Autodesk Inventor part; units mm, degrees
ref_plane "YZ Plane" through (0, 0, 0) normal (1, 0, 0) x (0, 1, 0)
ref_plane "XZ Plane" through (0, 0, 0) normal (0, 1, 0) x (-1, 0, 0)
ref_plane "XY Plane" through (0, 0, 0) normal (0, 0, 1) x (1, 0, 0)
sketch "Sketch1" plane through (0, 0, 0) normal (0, 1, 0) x (-1, 0, 0)
  arc A0 (27.5033, -3.6329) -> (24.5033, -6.6329) centre (27.5033, -6.6329) ccw
  arc A1 (28.5033, -3.6329) -> (28.5033, 4.3671) centre (28.5033, 0.3671) ccw
  line L0 (27.5033, -3.6329) -> (28.5033, -3.6329)
  line L1 (28.5033, 4.3671) -> (27.5033, 4.3671)
  arc A2 (24.5033, 7.3671) -> (27.5033, 4.3671) centre (27.5033, 7.3671) ccw
  line L2 (24.5033, 18.9671) -> (24.5033, 7.3671)
  line L3 (-28.2967, 18.9671) -> (24.5033, 18.9671)
  line L4 (-28.2967, 7.3671) -> (-28.2967, 18.9671)
  arc A3 (-31.2967, 4.3671) -> (-28.2967, 7.3671) centre (-31.2967, 7.3671) ccw
  line L5 (-31.2967, 4.3671) -> (-32.2967, 4.3671)
  arc A4 (-32.2967, 4.3671) -> (-32.2967, -3.6329) centre (-32.2967, 0.3671) ccw
  line L6 (-32.2967, -3.6329) -> (-31.2967, -3.6329)
  arc A5 (-28.2967, -6.6329) -> (-31.2967, -3.6329) centre (-31.2967, -6.6329) ccw
  line L7 (-28.2967, -18.2329) -> (-28.2967, -6.6329)
  line L8 (24.5033, -18.2329) -> (-28.2967, -18.2329)
  line L9 (24.5033, -6.6329) -> (24.5033, -18.2329)
  circle A6 centre (28.5033, 0.3671) radius 1.6
  circle A7 centre (-32.2967, 0.3671) radius 1.6
  circle A8 centre (-1.8967, 9.6671) radius 2.25
  circle A9 centre (15.2033, 9.6671) radius 2.25
  circle A10 centre (15.2033, -8.9329) radius 2.25
  circle A11 centre (-1.8967, -8.9329) radius 2.25
  circle A12 centre (-18.9967, -8.9329) radius 2.25
  circle A13 centre (-18.9967, 9.6671) radius 2.25
  point P0 (0, 0)
extrude "Extrusion1" add sketch "Sketch1" along normal blind 2.5
sketch "Sketch2" plane through (0, 2.5, 0) normal (0, 1, 0) x (1, 0, 0)
  line L0 (-12.6033, -12.2671) -> (-17.8033, -12.2671) construction
  line L1 (-17.8033, -12.2671) -> (-17.8033, -7.0671) construction
  line L2 (-17.8033, -7.0671) -> (-12.6033, -7.0671) construction
  line L3 (-12.6033, -7.0671) -> (-12.6033, -12.2671) construction
  circle A0 centre (-15.2033, -9.6671) radius 2.25 construction
  line L4 (-12.6033, -12.2671) -> (-17.8033, -7.0671) construction
  line L5 (-17.8033, -12.2671) -> (-12.6033, -7.0671) construction
  circle A1 centre (-17.8033, -7.0671) radius 0.75
  circle A2 centre (-12.6033, -12.2671) radius 0.75
  circle A3 centre (-17.8033, 11.5329) radius 0.75
  circle A4 centre (-12.6033, 6.3329) radius 0.75
  circle A5 centre (-0.7033, -7.0671) radius 0.75
  circle A6 centre (4.4967, -12.2671) radius 0.75
  circle A7 centre (-0.7033, 11.5329) radius 0.75
  circle A8 centre (4.4967, 6.3329) radius 0.75
  circle A9 centre (16.3967, -7.0671) radius 0.75
  circle A10 centre (21.5967, -12.2671) radius 0.75
  circle A11 centre (16.3967, 11.5329) radius 0.75
  circle A12 centre (21.5967, 6.3329) radius 0.75
  point P0 (0, 0)
  dimension "d2" = 1.5
  dimension "d3" = 1.5
  dimension "d6" = 18.6
  dimension "d9" = 17.1
  dimension "d14" = 5.2
  dimension "d15" = 5.2
extrude "Extrusion2" cut sketch "Sketch2" against normal through all
equation "\"d3\" = d2"
Design review of the part built by this model. Coordinates are the model's own, in mm. Round coordinates to 2 decimals unless told otherwise and drop trailing zeros. Order: outer loops, then holes, each group sorted by start corner. A loop starts at its lowest first (then second) coordinate and runs counter-clockwise, first axis right, second up. Notation, with made-up numbers: (-15.5, -27) - (-9.5, -27) arc R20 ccw to (-9.5, 12) - close; hole circle Ø2 at (83.25, 31). An arc over 180 degrees is marked (long way). One line per question, with ' | ' between items.
Item 1: Take a section at D-D, the plane z = -2. Write out the cut boundary in (x, y), then the cut area to 3 significant figures.
Checks:
outline: (-31.73, 0) - (35.52, 0) - (35.52, 2.5) - (-31.73, 2.5) - close | area: 168 mm²
Item 2: Take a section at B-B, the plane z = -10. Write out the cut boundary in (x, y).
Checks:
outline: (-24.5, 0) - (-17.18, 0) - (-17.18, 2.5) - (-24.5, 2.5) - close; (-13.22, 0) - (-0.08, 0) - (-0.08, 2.5) - (-13.22, 2.5) - close; (3.88, 0) - (17.02, 0) - (17.02, 2.5) - (3.88, 2.5) - close; (20.98, 0) - (28.3, 0) - (28.3, 2.5) - (20.98, 2.5) - close
Item 3: Draft analysis for pull direction Z (two halves, no side actions). For faces 1 (the face through (2, 0, 1)), 2 (the face through (29.2, 1.23, -4.49)), 3 (the face through (-12.77, 1.27, -5.6)), 4 (the face through (22.29, 1.27, -6.05)), state which applies: +Z half, -Z half, draft (parallel to the pull), parting line (faces both ways), or undercut.
Checks:
face 1: draft | face 2: -Z half | face 3: undercut | face 4: undercut
Item 4: Take a section at C-C, the plane y = 0.6. Give the number of separate pieces and of enclosed holes in the cut face, then the cut area to 3 significant figures.
Checks:
separate pieces: 1 | enclosed holes: 20 | area: 1,950 mm²
Item 5: Wall thickness on line 1 (Z direction, x = 2, y = 1.4); line 2 (X direction, y = 0.3, z = 9.5); line 3 (X direction, y = 1.5, z = 1): over which ranges is each line inside the solid? List them lowest first. Write a range as [from, to].
Checks:
line 1: [-18.23, -11.18], [-6.69, 7.42], [11.91, 18.97] | line 2: [-24.5, -17.45], [-12.96, -0.35], [4.14, 16.75], [21.24, 28.3] | line 3: [-32.45, -29.97], [-27.03, 30.83], [33.77, 36.25]
Item 6: Take a section at A-A, the plane x = 1. Write out the cut boundary in (y, z), then the cut area to 3 significant figures.
Checks:
outline: (0, -18.23) - (2.5, -18.23) - (2.5, -11) - (0, -11) - close; (0, -6.87) - (2.5, -6.87) - (2.5, 7.6) - (0, 7.6) - close; (0, 11.73) - (2.5, 11.73) - (2.5, 18.97) - (0, 18.97) - close | area: 72.4 mm²
Item 7: For P1, Ø0.8, axis at x = 31.5, y = 1, coming from the -Z side; P2, Ø2.5, axis at x = -28.5, z = 0.37, coming from the +Y side; P3, Ø1, axis at y = 1.5, z = -0.5, coming from the -X side, all flat-tipped, find the tip position at first contact; note any pin that passes through.
Checks:
P1: z = -3.64 | P2: through | P3: x = -32.49
